Could you check a few things on this drawing? It's one solid part, dimensions in mm from its lowest x, y, z. A direction names the side the tool comes from. Coordinates: 2 decimals unless noted, no trailing zeros. Write each loop counter-clockwise with the first axis right and the second up, starting at its lowest first coordinate (ties: lowest second). Pieces come first, ordered by that corner, then holes.
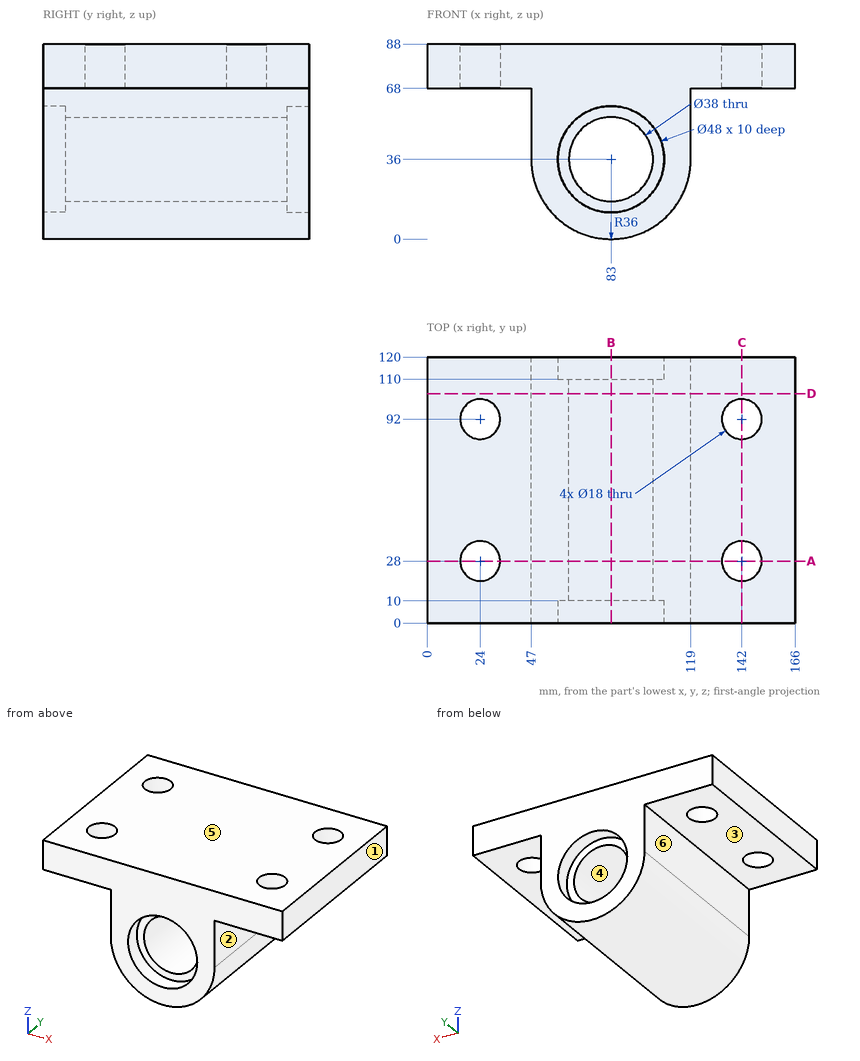
1) Imagine slicing it at A-A on y = 28. Please give me the cut outline in (x, z).
Values follow:
outline: (0, 68) - (15, 68) - (15, 88) - (0, 88) - close; (33, 68) - (47, 68) - (47, 36) arc R36 ccw to (119, 36) - (119, 68) - (133, 68) - (133, 88) - (33, 88) - close; (151, 68) - (166, 68) - (166, 88) - (151, 88) - close; hole circle Ø38 at (83, 36)
2) We'd pull the mould along Z, two halves only. Please class the marked faces 4, 5 and 6: pulls with the +Z half, pulls with the -Z half, needs draft (parallel to the pull), parting line crosses it, or undercut.
Values follow:
face 4: undercut
face 5: pulls with the +Z half
face 6: needs draft
3) On a 3-axis mill with a long thin cutter (end or side, diameter ignored), from which of +Z, -Z, +X, -X, +Y, -Y can I reach the whole of each face in a straight line? I mean the marked faces 1, 2 and 3. Say none if no direction works.
Values follow:
face 1: +Z, -Z, +X, +Y, -Y
face 2: -Z, +X, +Y, -Y
face 3: -Z, -X, +Y, -Y
4) Imagine slicing it at C-C on x = 142. Please give me the cut outline in (y, z).
Values follow:
outline: (0, 68) - (19, 68) - (19, 88) - (0, 88) - close; (37, 68) - (83, 68) - (83, 88) - (37, 88) - close; (101, 68) - (120, 68) - (120, 88) - (101, 88) - close
5) Imagine slicing it at B-B on x = 83. Please give me the cut outline in (y, z).
Values follow:
outline: (0, 0) - (120, 0) - (120, 12) - (110, 12) - (110, 17) - (10, 17) - (10, 12) - (0, 12) - close; (0, 60) - (10, 60) - (10, 55) - (110, 55) - (110, 60) - (120, 60) - (120, 88) - (0, 88) - close
6) Will these pins go through, and if not, where does the flat tip stop? pin 1 (4 mm diameter, centred on y = 90.5, z = 19.5, fed in from -X); pin 2 (1 mm diameter, centred on x = 85.5, y = 58, fed in from -Z); pin 3 (23.5 mm diameter, centred on x = 16.5, y = 61.5, fed in from -Z).
Values follow:
pin 1: stops at x = 50.05
pin 2: stops at z = 0.06
pin 3: stops at z = 68
7) I need wall thicknesses on probe 1 along Y at (x, z) = (24, 79.25); probe 2 along Z at (x, y) = (83, 31); probe 3 along Z at (x, y) = (153, 101). Which ranges of each line are inside material? Lowest first, please.
Values follow:
probe 1: y = 0 to 19, 37 to 83, 101 to 120
probe 2: z = 0 to 17, 55 to 88
probe 3: z = 68 to 88
8) Imagine slicing it at D-D on y = 103.5. Please give me the cut outline in (x, z), then the cut area to 3 significant figures.
Values follow:
outline: (0, 68) - (47, 68) - (47, 36) arc R36 ccw to (119, 36) - (119, 68) - (166, 68) - (166, 88) - (0, 88) - close; hole circle Ø38 at (83, 36)
area: 6,530 mm2
